```python
from build123d import *

# Parameters (mm, degrees)
F1_DEPTH  = 12.7
F3_DEPTH  = 38.1
F5_DEPTH  = 25.4
F7_DEPTH  = 12.7
F9_DEPTH  = 12.7
F10_R     = 3.96875
F11_DEPTH = 25.4
F12_DEPTH = 82.551
F13_R     = 9.525
F14_R     = 6.35


# Not quite as in the source:
# - a length typed as a fraction of an inch, garbled in the dataset ("3 / 203.2 mm" for 3/8 in), is restored


with BuildPart() as f1:
    # F0 (on Top) → F1 (new body)
    with BuildSketch(Plane.XY):
        with BuildLine():
            Line((-38.1, -38.1), (38.1, -38.1))
            ThreePointArc((38.1, -38.1), (76.2, 0), (38.1, 38.1))
            Line((38.1, 38.1), (-38.1, 38.1))
            ThreePointArc((-38.1, 38.1), (-76.2, 0), (-38.1, -38.1))
        make_face()
    extrude(amount=F1_DEPTH)

    # F2 (on Right) → F3 (join, symmetric)
    with BuildSketch(Plane.YZ):
        Polygon((6.4445460903, 82.55), (0, 82.55), (-6.2554539097, 82.55), (-22.225, 82.55), (-22.225, 69.85), (-6.2554539097, 69.85), (-6.2554539097, 0), (6.4445460903, 0), (6.4445460903, 69.85), (22.225, 69.85), (22.225, 82.55), align=None)
    extrude(amount=F3_DEPTH, both=True)

    # F4 (on face) → F5 (cut)
    with BuildSketch(Plane.XZ.offset(6.2554539097)):
        with BuildLine():
            Line((7.9375, 69.85), (-7.9375, 69.85))
            ThreePointArc((-7.9375, 69.85), (0, 61.9125), (7.9375, 69.85))
        make_face()
    extrude(amount=-F5_DEPTH, mode=Mode.SUBTRACT)

    # F6 (on face) → F7 (join)
    with BuildSketch(Plane.YZ.offset(38.1)):
        Polygon((-28.575, 12.7), (28.575, 12.7), (22.225, 69.85), (-22.225, 69.85), align=None)
    extrude(amount=-F7_DEPTH)

    # F8 (on face) → F9 (join)
    with BuildSketch(Plane(origin=(-38.1, 0, 0), x_dir=(0, -1, 0), z_dir=(-1, 0, 0))):
        Polygon((-22.225, 69.85), (-28.575, 12.6521781883), (28.575, 12.6521781883), (22.225, 69.85), align=None)
    extrude(amount=-F9_DEPTH)

    # F10 (on face) → F11 (cut)
    with BuildSketch(Plane.XY.offset(82.55)):
        with Locations((0, 14.2875)):
            Circle(F10_R)
        with Locations((0, -14.2875)):
            Circle(F10_R)
    extrude(amount=-F11_DEPTH, mode=Mode.SUBTRACT)

    # F10 (on face) → F12 (cut, through all)
    with BuildSketch(Plane.XY.offset(82.55)):
        with Locations((-57.15, 0)):
            Circle(F10_R)
        with Locations((57.15, 0)):
            Circle(F10_R)
    extrude(amount=-F12_DEPTH, mode=Mode.SUBTRACT)

    # F13
    f13_edges = [f1.edges().sort_by_distance(p)[0] for p in [
        (31.75, -28.575, 12.7),
        (31.75, 28.575, 12.7),
        (-31.75, -28.569691, 12.7),
        (-31.75, 28.569691, 12.7),
    ]]
    fillet(f13_edges, radius=F13_R)

    # F14
    f14_edges = [f1.edges().sort_by_distance(p)[0] for p in [
        (0, 6.444546, 12.7),
        (0, -6.255454, 12.7),
        (-16.66875, -6.255454, 69.85),
        (16.66875, -6.255454, 69.85),
        (-16.66875, 6.444546, 69.85),
        (16.66875, 6.444546, 69.85),
        (38.1, 0, 12.7),
        (-38.1, 0, 12.7),
        (-25.4, 6.444546, 41.275),
        (25.4, 6.444546, 41.275),
        (-25.4, -6.255454, 41.275),
        (25.4, -6.255454, 41.275),
    ]]
    fillet(f14_edges, radius=F14_R)


solid = f1.part
```
Could you check a few things on this model? Use its own coordinates, in mm. A direction names the side the tool comes from. Round coordinates to 2 decimals unless told otherwise and drop trailing zeros. Write each loop counter-clockwise with the first axis right and the second up, starting at its lowest first coordinate (ties: lowest second). Pieces come first, ordered by that corner, then holes. Notation, with made-up numbers: M 33,-37.75 L 75,-37.75 A24 cw 75,-13.75 Z; hole C 35,86.5 d10. An arc over 180 degrees is marked long. Answer in a Markdown table with one row per item. Add a question column.
Q1. If we mould it in two halves opening along X, with no side actions, what happens to faces 4 (the cylindrical face through (-40.01, -0.52, 14.51)), 5 (the cylindrical face through (15.226, 8.354, 68.039)), 6 (the cylindrical face through (-32.67, -30.82, 15.06))? For each: +X half, -X half, draft (parallel to the pull), parting line (faces both ways), or undercut.
Q2. Imagine slicing it at A-A (x = 0). Give the number of separate pieces and of enclosed holes in the cut face, then the cut area to 3 significant figures.
Q3. If I drill on line 1 (Y direction, x = 0, z = 73) (3 decimals); line 2 (Z direction, x = -21, y = 16); line 3 (X direction, y = 15, z = 51), over which ranges is the centre line in solid material (lowest first)? Write a range as from..to.
Q4. On a 3-axis mill with a long thin cutter (end or side, diameter ignored), from which of +Z, -Z, +X, -X, +Y, -Y can I reach the whole of each face in a straight line? I mean faces 1 (the flat face through (-25.4, 20, 42)), 2 (the flat face through (1, 22.225, 76)), 3 (the flat face through (-25.4, -19, 42)). Say none if no direction works.
Q5. Will these pins go through, and if not, where does the flat tip stop? pin 1 Ø19.5 at (y, z) = (-25.5, 34.5) entering from -X; pin 2 Ø12 at (y, z) = (-23, 51.5) entering from +X; pin 3 Ø4 at (x, z) = (16.5, 74.5) entering from -Y (3 decimals).
Q6. Imagine slicing it at D-D (z = 10). Please give me the cut outline in (x, y).
Q7. Imagine slicing it at C-C (z = 67.5). Please give me the cut outline in (x, y), then the cut area to 3 significant figures.
Values:
| question | item | result |
|---|---|---|
| 1 | face 4 | -X half |
| 1 | face 5 | undercut |
| 1 | face 6 | draft |
| 2 | separate pieces | 4 |
| 2 | enclosed holes | 0 |
| 2 | area | 1,970 mm^2 |
| 3 | line 1 | -22.225..-18.256, -10.319..10.319, 18.256..22.225 |
| 3 | line 2 | 0..12.7, 69.85..82.55 |
| 3 | line 3 | -38.1..-25.4, 25.4..38.1 |
| 4 | face 1 | +Y |
| 4 | face 2 | +Z, +X, -X, +Y |
| 4 | face 3 | -Y |
| 5 | pin 1 | x = -38.1 |
| 5 | pin 2 | x = 38.1 |
| 5 | pin 3 | y = -22.225 |
| 6 | outline | M -38.1,-38.1 L 38.1,-38.1 A38.1 ccw 38.1,38.1 L -38.1,38.1 A38.1 ccw Z; hole C -57.15,0 d7.94; hole C 57.15,0 d7.94 |
| 7 | outline | M -38.1,-22.49 L -25.4,-22.49 L -25.4,-12.61 A6.35 cw -23.05,-7.67 L -7.58,-7.67 L -7.58,7.86 L -23.05,7.86 A6.35 cw -25.4,12.79 L -25.4,22.49 L -38.1,22.49 Z; M 7.58,-7.67 L 23.05,-7.67 A6.35 cw 25.4,-12.61 L 25.4,-22.49 L 38.1,-22.49 L 38.1,22.49 L 25.4,22.49 L 25.4,12.79 A6.35 cw 23.05,7.86 L 7.58,7.86 Z |
| 7 | area | 1,710 mm^2 |
